Can you work these out from the model? Positions are in its coordinate system, mm. Give positions to 0.01 mm unless a question says otherwise; leave off trailing zeros. Order: outer loops, then holes, each group sorted by start corner. A loop starts at its lowest first (then second) coordinate and runs counter-clockwise, first axis right, second up. Notation, with made-up numbers: (-25, 49) -> (-18, 49) arc R19 ccw to (-18, 53) -> close; hole circle Ø3 at (82.5, 9.5). An arc over 180 degrees is marked (long way). Answer as a JSON object with one key per item and string values.
```python
from build123d import *

# Parameters (mm, degrees)
CONG_1_R                = 0.1
CHANFREIN1_SIZE         = 0.5
ESQUISSE4_W             = 0.574782946
ESQUISSE4_H             = 1.352018642
ENL_V_MAT_EXTRU_1_DEPTH = 10


with BuildPart() as part:
    # Esquisse1 → Révolution1 (revolve)
    with BuildSketch(Plane(origin=(0, 0, 0), x_dir=(1, 0, 0), z_dir=(0, 1, 0))):
        with BuildLine():
            Line((0, 0), (0, 6.5))
            Line((0, 6.5), (-1, 6.5))
            add(Edge.make_bspline(
                [(-1, 6.5), (0, 7), (2, 7)],
                knots=[0, 0, 0, 1, 1, 1], degree=2))
            Line((2, 7), (2, 0))
            Line((2, 0), (0, 0))
        make_face()
    revolve(axis=Axis((2, 0, -7), (0, 0, 1)))

    # Congé1
    cong_1_edges = [part.edges().sort_by_distance(p)[0] for p in [
        (5, 0, -6.5),
    ]]
    fillet(cong_1_edges, radius=CONG_1_R)

    # Chanfrein1
    chanfrein1_edges = [part.edges().sort_by_distance(p)[0] for p in [
        (4, 0, 0),
    ]]
    chamfer(chanfrein1_edges, length=CHANFREIN1_SIZE)

    # Esquisse4 → Enlèv. mat.-Extru.1 (cut, symmetric)
    with BuildSketch(Plane(origin=(0.478013725, -0.852953884, 0), x_dir=(-0.8723492061003342, -0.4888832811787661, 0), z_dir=(-0.48888328117876617, 0.8723492061003343, 0))):
        with Locations((-1.744698412, -7.456425035)):
            Rectangle(ESQUISSE4_W, ESQUISSE4_H)
    extrude(amount=ENL_V_MAT_EXTRU_1_DEPTH, both=True, mode=Mode.SUBTRACT)


solid = part.part
```
1. If we section it at A-A on z = -4: Please give me the cut outline in (x, y).
Worked answers:
{"outline": "circle Ø4 at (2, 0)"}
2. Will this pin go through, and if not, where does the flat tip stop? pin 1 Ø2 at (x, z) = (1, -3.5) entering from -Y.
Worked answers:
{"pin 1": "y = -2"}
3. Please list where these lines run through material, in increasing order: L1, parallel to Z at x = 1.5, y = 1.1; L2, parallel to X at y = -1.5, z = -3.5; L3, parallel to Y at x = 3.8, z = -5.5.
Worked answers:
{"L1": "-6.78 to 0", "L2": "0.68 to 3.32", "L3": "-0.87 to 0.87"}
4. If we mould it in two halves opening along Y, with no side actions, what happens to faces 1 (the face through (2, 0, -6.78)), 2 (the face through (2, 2, -4)), 3 (the face through (2, 0, 0))? For each: +Y half, -Y half, draft (parallel to the pull), parting line (faces both ways), or undercut.
Worked answers:
{"face 1": "undercut", "face 2": "parting line", "face 3": "draft"}
